Can you work these out from the model? Positions are in its coordinate system, mm. A direction names the side the tool comes from. Give positions to 0.01 mm unless a question says otherwise; leave off trailing zeros. Order: outer loops, then holes, each group sorted by start corner. A loop starts at its lowest first (then second) coordinate and runs counter-clockwise, first axis right, second up. Notation, with made-up numbers: (54, 34) -> (86, 34) arc R12 ccw to (86, 53) -> close; hole circle Ø8 at (5, 71). An arc over 180 degrees is marked (long way). Answer as a JSON object with one key per item and string values.
```python
from build123d import *

# Parameters (mm, degrees)
F1_DEPTH = 6.35
F2_R     = 1.35255
F3_DEPTH = 4.7625


with BuildPart() as f1:
    # F0 (on Top) → F1 (new body)
    with BuildSketch(Plane.XY):
        Polygon((0, 1.5875), (0, 0), (1.5875, 0), (1.5875, -3.175), (0, -3.175), (0, -4.7625), (1.5875, -4.7625), (1.5875, -7.9375), (0, -7.9375), (0, -10.9855), (-25.69911, -10.9855), (-25.69911, 1.5875), (-32.04911, 1.5875), (-32.04911, 0), (-30.46161, 0), (-30.46161, -3.175), (-32.04911, -3.175), (-32.04911, -4.7625), (-30.46161, -4.7625), (-30.46161, -7.9375), (-32.04911, -7.9375), (-32.04911, -14.1605), (6.35, -14.1605), (6.35, 1.5875), align=None)
    extrude(amount=F1_DEPTH)

    # F2 (on face) → F3 (cut)
    with BuildSketch(Plane.XZ.offset(14.1605)):
        with Locations((-28.87411, 3.175)):
            Circle(F2_R)
        with Locations((3.175, 3.175)):
            Circle(F2_R)
    extrude(amount=-F3_DEPTH, mode=Mode.SUBTRACT)


solid = f1.part
```
1. For faces 4 (the face through (1.588, -6, 3)), 5 (the face through (-30.225, -11.813, 3.234)), 6 (the face through (0, -9, 3)), 7 (the face through (-31, -4.762, 3)), which set-ups out of +Z, -Z, +X, -X, +Y, -Y let a thin tool reach every point of the face, with its end or its side?
Worked answers:
{"face 4": "+Z, -Z", "face 5": "-Y", "face 6": "+Z, -Z, +Y", "face 7": "+Z, -Z, -X"}
2. Will these pins go through, and if not, where does the flat tip stop? pin 1 Ø1.5 at (x, y) = (-23.5, -6.5) entering from -Z; pin 2 Ø3 at (x, z) = (-3.5, 2.5) entering from +Y; pin 3 Ø2.5 at (y, z) = (-1.5, 2.5) entering from -X.
Worked answers:
{"pin 1": "through", "pin 2": "y = -10.99", "pin 3": "x = -30.46"}
3. If we mould it in two halves opening along Z, with no side actions, what happens to faces 1 (the face through (-13, -10.986, 3)), 2 (the face through (-17.4, -11.4, 0)), 3 (the face through (-29, -9.398, 3))? For each: +Z half, -Z half, draft (parallel to the pull), parting line (faces both ways), or undercut.
Worked answers:
{"face 1": "draft", "face 2": "-Z half", "face 3": "undercut"}
4. Please list where these lines run through material, in increasing order: L1, parallel to X at y = -10.5, z = 3.25; L2, parallel to X at y = -11.5, z = 3.25; L3, parallel to X at y = -1.75, z = 2.
Worked answers:
{"L1": "-32.05 to -30.22, -27.52 to -25.7, 0 to 1.82, 4.53 to 6.35", "L2": "-32.05 to -30.22, -27.52 to 1.82, 4.53 to 6.35", "L3": "-30.46 to -25.7, 1.59 to 6.35"}
5. If we section it at A-A on y = -5.5: Please give me the cut outline in (x, z), then the cut area to 3 significant figures.
Worked answers:
{"outline": "(-30.46, 0) -> (-25.7, 0) -> (-25.7, 6.35) -> (-30.46, 6.35) -> close; (1.59, 0) -> (6.35, 0) -> (6.35, 6.35) -> (1.59, 6.35) -> close", "area": "60.5 mm²"}
6. If we section it at D-D on y = -12.25: Please give me the cut outline in (x, z) (3 decimals).
Worked answers:
{"outline": "(-32.049, 0) -> (6.35, 0) -> (6.35, 6.35) -> (-32.049, 6.35) -> close; hole circle Ø2.705 at (-28.874, 3.175); hole circle Ø2.705 at (3.175, 3.175)"}
7. If we section it at B-B on x = 1: Count the separate pieces of the cut face and the enclosed holes in it, then the cut area to 3 significant figures.
Worked answers:
{"separate pieces": "3", "enclosed holes": "0", "area": "59.7 mm²"}
